```python
from build123d import *

# Parameters (mm, degrees)
BOSS_EXTRUDE1_DEPTH = 42
SKETCH2_R           = 15
CUT_EXTRUDE1_DEPTH  = 74
SKETCH3_W           = 20
SKETCH3_H           = 12
CUT_EXTRUDE4_DEPTH  = 74
SKETCH4_W           = 30
SKETCH4_H           = 30
BOSS_EXTRUDE2_DEPTH = 20
SKETCH5_R           = 6
CUT_EXTRUDE5_DEPTH  = 30
SKETCH6_R           = 10
CUT_EXTRUDE6_DEPTH  = 40


with BuildPart() as part:
    # Sketch1 → Boss-Extrude1 (new body)
    with BuildSketch(Plane.XY):
        Polygon((0, 0), (74, 0), (74, 28), (34, 28), (0, 20), align=None)
    extrude(amount=-BOSS_EXTRUDE1_DEPTH)

    # Sketch2 → Cut-Extrude1 (cut)
    with BuildSketch(Plane.ZY):
        with Locations((-21, 0)):
            Circle(SKETCH2_R)
    extrude(amount=-CUT_EXTRUDE1_DEPTH, mode=Mode.SUBTRACT)

    # Sketch3 → Cut-Extrude4 (cut)
    with BuildSketch(Plane(origin=(-4.459016393, 18.950819672, 0), x_dir=(0.973417168, 0.229039334, 0), z_dir=(-0.229039334, 0.973417168, 0))):
        with Locations((21.580786675, 21)):
            Rectangle(SKETCH3_W, SKETCH3_H)
    extrude(amount=-CUT_EXTRUDE4_DEPTH, mode=Mode.SUBTRACT)

    # Sketch4 → Boss-Extrude2 (add)
    with BuildSketch(Plane(origin=(0, 28, 0), x_dir=(1, 0, 0), z_dir=(0, 1, 0))):
        with Locations((54, 21)):
            Rectangle(SKETCH4_W, SKETCH4_H)
    extrude(amount=BOSS_EXTRUDE2_DEPTH)

    # Sketch5 → Cut-Extrude5 (cut)
    with BuildSketch(Plane.ZY.offset(-39)):
        with Locations((-21, 38)):
            Circle(SKETCH5_R)
    extrude(amount=-CUT_EXTRUDE5_DEPTH, mode=Mode.SUBTRACT)

    # Sketch6 → Cut-Extrude6 (cut)
    with BuildSketch(Plane(origin=(0, 48, 0), x_dir=(1, 0, 0), z_dir=(0, 1, 0))):
        with Locations((54, 21)):
            Circle(SKETCH6_R)
    extrude(amount=-CUT_EXTRUDE6_DEPTH, mode=Mode.SUBTRACT)


solid = part.part
```
CAD build for the part. Positions are in the model's coordinates, mm. A direction names the side the tool comes from. Coordinates: 2 decimals unless noted, no trailing zeros. Write each loop counter-clockwise with the first axis right and the second up, starting at its lowest first coordinate (ties: lowest second). Pieces come first, ordered by that corner, then holes.
(1) Cut at A-A, the plane x = 54. List the corners of the cut face in (y, z).
(2) Cut at B-B, the plane y = 38. List the corners of the cut face in (x, z).
(3) Flat gauge pins, fed straight in: pin 1 (10 mm diameter, centred on y = 36, z = -19.5, fed in from -X); pin 2 (1.5 mm diameter, centred on x = 56, z = -8, fed in from -Y); pin 3 (1.5 mm diameter, centred on x = 62, z = -8.5, fed in from -Y). Where does each tip first touch, or does it go through?
(4) Cut at D-D, the plane x = 40.5. List the corners of the cut face in (y, z).
(5) Drill centre lines: probe 1 along Z at (x, y) = (44.5, 38); probe 2 along Y at (x, z) = (66, -21); probe 3 along X at (y, z) = (17.5, -25). Where is each one in solid material? Low to high.
(6) Two-plate mould, pull along X, no slides. Class faces 1 (the face through (18, 19, -15)), 2 (the face through (36, 14, -42)), 3 (the face through (74, 17, -21)): +X half, -X half, draft (parallel to the pull), parting line (faces both ways), or undercut.
(7) Cut at C-C, the plane z = -18. List the corners of the cut face in (x, y), and give its area (3 significant figures).
(8) 3-axis set-ups, long thin cutter, end or side, ignore diameter. For faces 4 (the face through (54, 38, -6)), 5 (the face through (69, 37.9, -27.5)), 6 (the face through (27.725, 20.053, -20.916)), 7 (the face through (44, 30, -21)), 8 (the face through (54, 38, -36)): which of +Z, -Z, +X, -X, +Y, -Y reach the whole face in a straight line?
Geometry says:
1. outline: (0, -42) - (28, -42) - (28, -36) - (48, -36) - (48, -31) - (11.18, -31) arc R15 cw to (0, -36) - close; (0, -6) arc R15 cw to (11.18, -11) - (48, -11) - (48, -6) - (28, -6) - (28, 0) - (0, 0) - close
2. outline: (39, -36) - (69, -36) - (69, -27) - (62, -27) arc R10 cw to (46, -27) - (39, -27) - close; (39, -15) - (46, -15) arc R10 cw to (62, -15) - (69, -15) - (69, -6) - (39, -6) - close
3. pin 1: stops at x = 39
3. pin 2: stops at y = 5.99
3. pin 3: stops at y = 7.03
4. outline: (0, -42) - (28, -42) - (28, -36) - (48, -36) - (48, -6) - (28, -6) - (28, 0) - (0, 0) - (0, -6) arc R15 cw to (0, -36) - close; hole circle Ø12 at (38, -21)
5. probe 1: z = -36 to -27, -15 to -6
5. probe 2: y = 15 to 32, 44 to 48
5. probe 3: x = 0 to 7.78, 28.33 to 44.83, 63.17 to 74
6. face 1: undercut
6. face 2: draft
6. face 3: +X half
7. outline: (0, 14.7) - (8.44, 14.7) - (6.81, 21.6) - (0, 20) - close; (26.28, 26.18) - (28.99, 14.7) - (44.46, 14.7) - (44.46, 32.8) - (39, 32.8) - (39, 28) - (34, 28) - close; (39, 43.2) - (44.46, 43.2) - (44.46, 48) - (39, 48) - close; (63.54, 14.7) - (74, 14.7) - (74, 28) - (69, 28) - (69, 32.8) - (63.54, 32.8) - close; (63.54, 43.2) - (69, 43.2) - (69, 48) - (63.54, 48) - close
7. area: 511 mm2
8. face 4: +Z, +X, -X, +Y
8. face 5: +Z, -Z, +X, +Y
8. face 6: -Y
8. face 7: +Y, -Y
8. face 8: -Z, +X, -X, +Y
